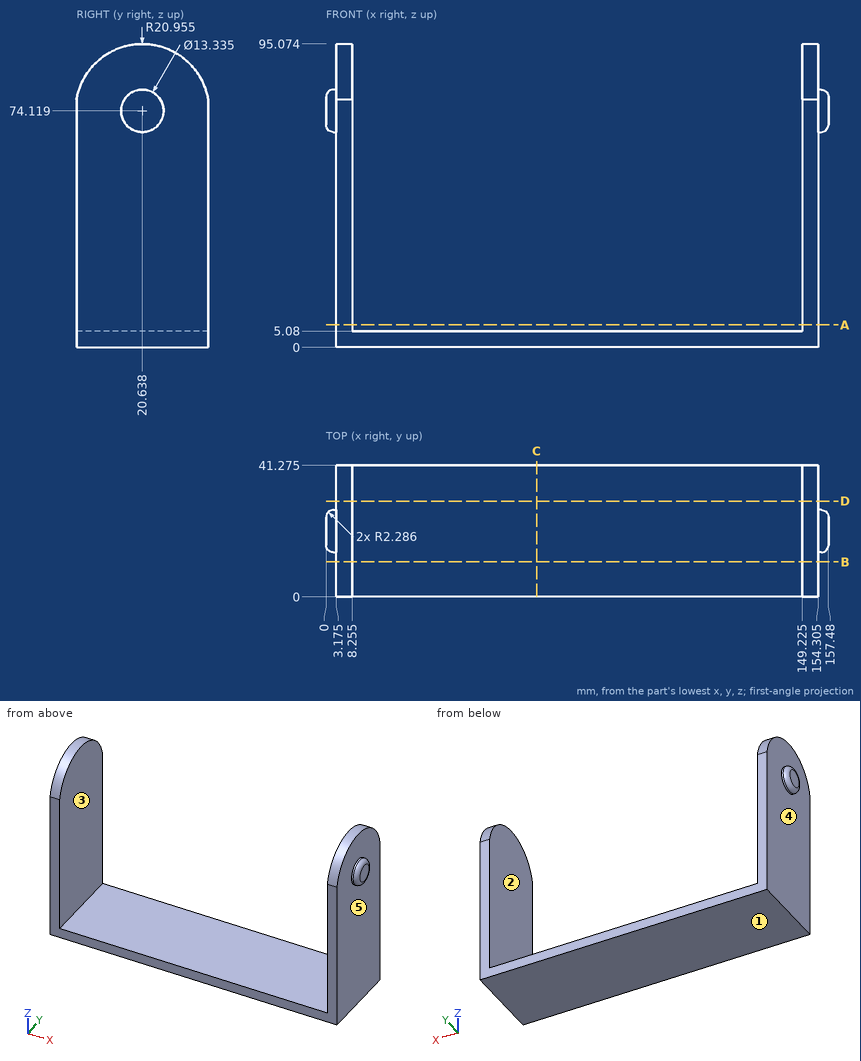
The figure shows three views and two pictorial views of one solid part (mm, origin at its lowest corner). Answer the questions. A direction names the side the tool comes from. Give positions to 0.01 mm unless a question says otherwise; leave off trailing zeros. Write each loop counter-clockwise with the first axis right and the second up, starting at its lowest first coordinate (ties: lowest second). Pieces come first, ordered by that corner, then holes. Notation, with made-up numbers: (28, 51) -> (60, 51) arc R20 cw to (60, 62) -> close; hole circle Ø9 at (78.25, -37). An arc over 180 degrees is marked (long way). Write each question's results on one line, items separated by ' | '.
1. Find section A-A on z = 7. Determine the outline of the cut face in (x, y) (1 decimal).
Data:
outline: (3.2, 0) -> (8.3, 0) -> (8.3, 41.3) -> (3.2, 41.3) -> close; (149.2, 0) -> (154.3, 0) -> (154.3, 41.3) -> (149.2, 41.3) -> close
2. A tool of negligible diameter and unlimited length cuts with its end or side. For the marked faces 1 and 2, from which of +Z, -Z, +X, -X, +Y, -Y can it reach the whole face along a straight path? Write none if from no direction.
Data:
face 1: -Z, +X, -X, +Y, -Y | face 2: +Z, +Y, -Y
3. Determine the mould class of the marked faces 3, 4 and 5 for opening direction X: +X half, -X half, draft (parallel to the pull), parting line (faces both ways), or undercut.
Data:
face 3: undercut | face 4: -X half | face 5: +X half
4. Find section B-B on y = 11. Determine the outline of the cut face in (x, z) (1 decimal), and give its area (3 significant figures).
Data:
outline: (3.2, 0) -> (154.3, 0) -> (154.3, 92.7) -> (149.2, 92.7) -> (149.2, 5.1) -> (8.3, 5.1) -> (8.3, 92.7) -> (3.2, 92.7) -> close | area: 1,660 mm^2
5. Find section D-D on y = 30. Determine the outline of the cut face in (x, z) (1 decimal), and give its area (3 significant figures).
Data:
outline: (3.2, 0) -> (154.3, 0) -> (154.3, 92.9) -> (149.2, 92.9) -> (149.2, 5.1) -> (8.3, 5.1) -> (8.3, 92.9) -> (3.2, 92.9) -> close | area: 1,660 mm^2
6. Straight lines are drawn through the part: L1, parallel to X at y = 11, z = 53 (1 decimal); L2, parallel to Z at x = 66.5, y = 17. For each, find the intervals that lie inside material, in ascending order.
Data:
L1: 3.2 to 8.3, 149.2 to 154.3 | L2: 0 to 5.08
7. Find section C-C on x = 66. Determine the outline of the cut face in (y, z) (1 decimal), and give its area (3 significant figures).
Data:
outline: (0, 0) -> (41.3, 0) -> (41.3, 5.1) -> (0, 5.1) -> close | area: 210 mm^2
8. Each of these flat-tipped pins is pushed along its axis until it touches: pin 1 Ø6 at (x, y) = (84, 25) entering from +Z; pin 2 Ø8 at (y, z) = (27.5, 51.5) entering from +X (1 decimal); pin 3 Ø20.5 at (y, z) = (18.5, 56.5) entering from -X (1 decimal). Where does it stop, or does it pass through?
Data:
pin 1: z = 5.08 | pin 2: x = 154.3 | pin 3: x = 3.2
